from build123d import *

# Parameters (mm, degrees)
F2_R      = 13.5
F2_R_2    = 10
F3_DEPTH  = 2
F4_DEPTH  = 25
F5_R      = 16.5
F6_DEPTH  = 10
F7_R      = 12.5
F8_DEPTH  = 9.5
F10_DEPTH = 7
F11_SIZE  = 0.5
F12_SIZE  = 1
F13_SIZE  = 0.8


with BuildPart() as f1:
    # F0 (on Front) → F1 (revolve)
    with BuildSketch(Plane.XZ):
        Polygon((0, 210), (0, 0), (26, 0), (26, 24), (22, 24), (22, 35), (45, 35), (45, 95), (50, 95), (50, 103), (42, 106.5), (42, 114.5), (50, 118), (50, 134), (49, 135), (25, 135), (25, 156.5), (24, 163), (24, 196), (25, 202.5), (25, 207.5), (22.5, 210), align=None)
    revolve(axis=Axis((0, 0, 105), (0, 0, 1)))

    # F2 (on face) → F3 (cut)
    with BuildSketch(Plane(origin=(0, 0, 0), x_dir=(1, 0, 0), z_dir=(0, 0, -1))):
        Circle(F2_R)
        Circle(F2_R_2, mode=Mode.SUBTRACT)
    extrude(amount=-F3_DEPTH, mode=Mode.SUBTRACT)

    # F2 (on face) → F4 (cut)
    with BuildSketch(Plane(origin=(0, 0, 0), x_dir=(1, 0, 0), z_dir=(0, 0, -1))):
        Circle(F2_R_2)
    extrude(amount=-F4_DEPTH, mode=Mode.SUBTRACT)

    # F5 (on face) → F6 (cut)
    with BuildSketch(Plane.XY.offset(210)):
        Circle(F5_R)
    extrude(amount=-F6_DEPTH, mode=Mode.SUBTRACT)

    # F7 (on face) → F8 (join)
    with BuildSketch(Plane.XY.offset(200)):
        Circle(F7_R)
    extrude(amount=F8_DEPTH)

    # F9 (on face) → F10 (cut)
    with BuildSketch(Plane.XY.offset(209.5)):
        with BuildLine():
            ThreePointArc((12.5, 0), (12.2307213882, 2.5805918554), (11.4344873081, 5.05))
            Line((11.4344873081, 5.05), (-11.4344873081, 5.05))
            ThreePointArc((-11.4344873081, 5.05), (-12.5, 0), (-11.4344873081, -5.05))
            Line((-11.4344873081, -5.05), (11.4344873081, -5.05))
            ThreePointArc((11.4344873081, -5.05), (12.2307213882, -2.5805918554), (12.5, 0))
        make_face()
    extrude(amount=-F10_DEPTH, mode=Mode.SUBTRACT)

    # F11
    f11_edges = [f1.edges().sort_by_distance(p)[0] for p in [
        (0, 5.05, 209.5),
        (0, 12.5, 209.5),
        (0, -12.5, 209.5),
        (0, -5.05, 209.5),
    ]]
    chamfer(f11_edges, length=F11_SIZE)

    # F12
    f12_edges = [f1.edges().sort_by_distance(p)[0] for p in [
        (-50, 0, 95),
    ]]
    chamfer(f12_edges, length=F12_SIZE)

    # F13
    f13_edges = [f1.edges().sort_by_distance(p)[0] for p in [
        (-26, 0, 24),
        (-26, 0, 0),
    ]]
    chamfer(f13_edges, length=F13_SIZE)


solid = f1.part
Check sheet for the modelled part. Datum: model origin and axes. Units: mm. A direction names the side the tool comes from. Give positions to 0.01 mm unless a question says otherwise; leave off trailing zeros. Write each loop counter-clockwise with the first axis right and the second up, starting at its lowest first coordinate (ties: lowest second). Pieces come first, ordered by that corner, then holes. Notation, with made-up numbers: (-9.75, 4.25) -> (20.25, 4.25) arc R23 ccw to (20.25, 20.25) -> close; hole circle Ø10 at (63.25, 32.5). An arc over 180 degrees is marked (long way). One line per item, written item: value. Start each with the question number.
Item 1: Gauge pin test, flat ends, axial feed: pin 1 (8 mm diameter, centred on x = 2.5, z = 64.5, fed in from +Y); pin 2 (5 mm diameter, centred on y = 28.5, z = 47.5, fed in from -X); pin 3 (2 mm diameter, centred on x = -21.5, z = 109, fed in from -Y); pin 4 (25 mm diameter, centred on x = -8, y = -12.5, fed in from +Z). Record the tip position at first contact, or that the pin passes through.
Item 2: Tool access check on faces 4 (the flat face through (-12, 12, 210)), 5 (the cylindrical face through (-20.633, -15.821, 12.157)), 6 (the flat face through (0, -8, 209.5)), 7 (the conical face through (-5.5, 42.1, 114.7)). Record the directions out of +Z, -Z, +X, -X, +Y, -Y that give a thin tool (end or side, any length) a straight path to the whole face; none if there is none.
Item 3: Section check A-A on z = 130. Record the cut outline in (x, y).
Item 4: Draft check along Z on faces 1 (the conical face through (11.097, -21.335, 162.684)), 2 (the flat face through (0, -5.05, 206)), 3 (the flat face through (0, 0, 25)). Enter one of: +Z half, -Z half, draft (parallel to the pull), parting line (faces both ways), or undercut.
Item 5: Material ranges on probe 1 along Y at (x, z) = (0, 203); probe 2 along Y at (x, z) = (0, 1.65); probe 3 along Y at (x, z) = (0, 19.75), recorded low to high. Write a range as from..to.
Item 6: Section check B-B on z = 177. Record the cut outline in (x, y), then the cut area to 3 significant figures.
Results list:
1. pin 1: y = 45
1. pin 2: x = -36.73
1. pin 3: y = -36.66
1. pin 4: z = 210
2. face 4: +Z, +X, -X, +Y, -Y
2. face 5: -Z
2. face 6: +Z
2. face 7: none
3. outline: circle Ø100 at (0, 0)
4. face 1: undercut
4. face 2: draft
4. face 3: -Z half
5. probe 1: -25..-16.5, -12.5..-5.05, 5.05..12.5, 16.5..25
5. probe 2: -26..-13.5, 13.5..26
5. probe 3: -26..-10, 10..26
6. outline: circle Ø48 at (0, 0)
6. area: 1,810 mm²
